from build123d import *

# Parameters (mm, degrees)
BOSS_EXTRUDE1_DEPTH = 13.2
CUT_EXTRUDE4_DEPTH  = 55.426464151
CUT_EXTRUDE5_DEPTH  = 55.426464151
SKETCH5_R           = 1.5
CUT_EXTRUDE6_DEPTH  = 55.426464151
SKETCH6_R           = 3
CUT_EXTRUDE7_DEPTH  = 2


with BuildPart() as part:
    # Sketch1 → Boss-Extrude1 (new body)
    with BuildSketch(Plane.XY):
        Polygon((0, 29.5), (6, 29.5), (6, 32), (36, 32), (36, 29.5), (42, 29.5), (42, 2.5), (36, 2.5), (36, 0), (6, 0), (6, 2.5), (0, 2.5), align=None)
    extrude(amount=BOSS_EXTRUDE1_DEPTH)

    # Sketch3 → Cut-Extrude4 (cut, through all)
    with BuildSketch(Plane(origin=(0, 0, 0), x_dir=(0, 0, -1), z_dir=(1, 0, 0))):
        Polygon((-2.4, 19.75), (0, 19.75), (0, 12.25), (-2.4, 12.25), (-3.4, 11.25), (-3.4, 7.5), (-8, 7.5), (-8, 24.5), (-3.4, 24.5), (-3.4, 20.75), align=None)
    extrude(amount=CUT_EXTRUDE4_DEPTH, mode=Mode.SUBTRACT)

    # Sketch4 → Cut-Extrude5 (cut, through all)
    with BuildSketch(Plane(origin=(0, 0, 0), x_dir=(0, 0, -1), z_dir=(1, 0, 0))):
        Polygon((-13.2, 24), (-12.9, 23.7), (-12.9, 8.3), (-13.2, 8), align=None)
        Polygon((0, 3), (-3, 0), (0, 0), align=None)
        Polygon((0, 32), (0, 29), (-3, 32), align=None)
        Polygon((-0.98, 12.25), (0, 9.75), (0, 12.25), align=None)
        Polygon((-0.98, 19.75), (0, 22.25), (0, 19.75), align=None)
    extrude(amount=CUT_EXTRUDE5_DEPTH, mode=Mode.SUBTRACT)

    # Sketch5 → Cut-Extrude6 (cut, through all)
    with BuildSketch(Plane.XY.offset(13.2)):
        with Locations((11, 28.5)):
            Circle(SKETCH5_R)
        with Locations((31, 28.5)):
            Circle(SKETCH5_R)
        with Locations((31, 3.5)):
            Circle(SKETCH5_R)
        with Locations((11, 3.5)):
            Circle(SKETCH5_R)
    extrude(amount=-CUT_EXTRUDE6_DEPTH, mode=Mode.SUBTRACT)

    # Sketch6 → Cut-Extrude7 (cut)
    with BuildSketch(Plane(origin=(0, 0, 0), x_dir=(-1, 0, 0), z_dir=(0, 0, -1))):
        with Locations((-31, 28.5)):
            Circle(SKETCH6_R)
        with Locations((-11, 28.5)):
            Circle(SKETCH6_R)
        with Locations((-11, 3.5)):
            Circle(SKETCH6_R)
        with Locations((-31, 3.5)):
            Circle(SKETCH6_R)
    extrude(amount=-CUT_EXTRUDE7_DEPTH, mode=Mode.SUBTRACT)


solid = part.part
Source: CAD feature listing. Evaluate the final solid. Frame: model axes, mm. A direction names the side the tool comes from. Give positions to 0.01 mm unless a question says otherwise; leave off trailing zeros. Write each loop counter-clockwise with the first axis right and the second up, starting at its lowest first coordinate (ties: lowest second). Pieces come first, ordered by that corner, then holes. Notation, with made-up numbers: M 87,2.25 L 95,2.25 A27 ccw 95,29.25 Z; hole C -22.75,36.5 d11. An arc over 180 degrees is marked long. Return JSON: item names as keys, results as strings. Group by question number.
1) Pin query (flat end, axial travel): P1, Ø3, axis at x = 39.5, z = 7, coming from the -Y side; P2, Ø2, axis at y = 31.5, z = 7, coming from the -X side; P3, Ø1.2, axis at y = 31.5, z = 7.5, coming from the +X side. Return the tip coordinate at first contact, or that it passes through.
2) Cut plane C-C, the plane z = 9.25. Output: boundary loops of the cut face in (x, y).
3) Pull-direction query (X, two-part tool) for faces 1 (the face through (29.5, 3.57, 7.68)), 2 (the face through (11.1, 25.5, 1)), 3 (the face through (36, 31, 7)), 4 (the face through (21, 26, 0)); classes: pulls with the +X half, pulls with the -X half, needs draft (parallel to the pull), parting line crosses it, or undercut.
4) Set-up query: faces 5 (the face through (39, 29.5, 7)), 6 (the face through (30, 5, 2)), 7 (the face through (21, 24.5, 6)), 8 (the face through (39, 2.5, 7)). Return all of +Z, -Z, +X, -X, +Y, -Y with unobstructed straight access to the full face (end or side cutting, diameter ignored); none if empty.
5) Material intervals for line 1 along X through (y, z) = (3.5, 1.05); line 2 along Y through (x, z) = (14.5, 5.5); line 3 along Y through (x, z) = (11, 5.75), sorted ascending. Write a range as [from, to].
6) Cut plane A-A, the plane z = 6.5. Output: boundary loops of the cut face in (x, y), plus the area to 3 significant figures.
7) Cut plane B-B, the plane y = 3.5. Output: boundary loops of the cut face in (x, z).
8) Cut plane D-D, the plane x = 11. Give the number of separate pieces and of enclosed holes in the cut face, plus the area to 3 significant figures.
Recorded:
{
 "1": {"P1": "stops at y = 2.5", "P2": "stops at x = 6", "P3": "stops at x = 36"},
 "2": {"outline": "M 0,2.5 L 6,2.5 L 6,0 L 36,0 L 36,2.5 L 42,2.5 L 42,29.5 L 36,29.5 L 36,32 L 6,32 L 6,29.5 L 0,29.5 Z; hole C 11,3.5 d3; hole C 11,28.5 d3; hole C 31,3.5 d3; hole C 31,28.5 d3"},
 "3": {"face 1": "undercut", "face 2": "undercut", "face 3": "pulls with the +X half", "face 4": "needs draft"},
 "4": {"face 5": "+Z, -Z, +X, +Y", "face 6": "-Z", "face 7": "+X, -X", "face 8": "+Z, -Z, +X, -Y"},
 "5": {"line 1": "x = [0, 8], [14, 28], [34, 42]", "line 2": "y = [0, 7.5], [24.5, 32]", "line 3": "y = [0, 2], [5, 7.5], [24.5, 27], [30, 32]"},
 "6": {"outline": "M 0,2.5 L 6,2.5 L 6,0 L 36,0 L 36,2.5 L 42,2.5 L 42,7.5 L 0,7.5 Z; M 0,24.5 L 42,24.5 L 42,29.5 L 36,29.5 L 36,32 L 6,32 L 6,29.5 L 0,29.5 Z; hole C 11,3.5 d3; hole C 11,28.5 d3; hole C 31,3.5 d3; hole C 31,28.5 d3", "area": "542 mm²"},
 "7": {"outline": "M 0,0 L 8,0 L 8,2 L 9.5,2 L 9.5,13.2 L 0,13.2 Z; M 12.5,2 L 14,2 L 14,0 L 28,0 L 28,2 L 29.5,2 L 29.5,13.2 L 12.5,13.2 Z; M 32.5,2 L 34,2 L 34,0 L 42,0 L 42,13.2 L 32.5,13.2 Z"},
 "8": {"separate pieces": "3", "enclosed holes": "0", "area": "216 mm²"}
}
